from build123d import *

# Parameters (mm, degrees)
F0_W     = 125
F0_H     = 100
F2_DEPTH = 63.5
F1_R     = 37.5
F3_DEPTH = 2.5
F5_DEPTH = 1
F6_R     = 1.5
F7_DEPTH = 20


# Not quite as in the source:
# - a feature names something its author has since deleted; it is built from what else it names


with BuildPart() as f2:
    # F0 (on Front) → F2 (new body)
    with BuildSketch(Plane.XZ):
        with Locations((0, 17.5)):
            Rectangle(F0_W, F0_H)
    extrude(amount=-F2_DEPTH)

    # F1 (on Front) → F3 (cut, symmetric)
    with BuildSketch(Plane.XZ):
        with Locations((-13.5, 22.6666666667)):
            Circle(F1_R)
    extrude(amount=F3_DEPTH, both=True, mode=Mode.SUBTRACT)

    # F4 (on face) → F5 (cut)
    with BuildSketch(Plane.XY.offset(67.5)):
        Polygon((51.0344103292, 5), (52.5, 5), (52.5, 7.5384757729), align=None)
        Polygon((46.0344103292, 5), (51.0344103292, 5), (52.5, 7.5384757729), (52.5, 16.1987298108), align=None)
        Polygon((36.0344103292, 5), (41.0344103292, 5), (52.5, 24.8589838486), (52.5, 33.5192378865), align=None)
        Polygon((26.0344103292, 5), (31.0344103292, 5), (52.5, 42.1794919243), (52.5, 50.8397459622), align=None)
        Polygon((16.0344103292, 5), (21.0344103292, 5), (52.5, 59.5), (47.5, 59.5), align=None)
        Polygon((-32.5, 59.5), (-52.5, 24.8589838486), (-52.5, 16.1987298108), (-27.5, 59.5), align=None)
        Polygon((6.0344103292, 5), (11.0344103292, 5), (42.5, 59.5), (37.5, 59.5), align=None)
        Polygon((-52.5, 42.1794919243), (-52.5, 33.5192378865), (-37.5, 59.5), (-42.5, 59.5), align=None)
        Polygon((-47.5, 59.5), (-52.5, 59.5), (-52.5, 50.8397459622), align=None)
        Polygon((-22.5, 59.5), (-52.5, 7.5384757729), (-52.5, 5), (-48.9655896708, 5), (-17.5, 59.5), align=None)
        Polygon((-3.9655896708, 5), (1.0344103292, 5), (32.5, 59.5), (27.5, 59.5), align=None)
        Polygon((-13.9655896708, 5), (-8.9655896708, 5), (22.5, 59.5), (17.5, 59.5), align=None)
        Polygon((-12.5, 59.5), (-43.9655896708, 5), (-38.9655896708, 5), (-7.5, 59.5), align=None)
        Polygon((-23.9655896708, 5), (-18.9655896708, 5), (12.5, 59.5), (7.5, 59.5), align=None)
        Polygon((-2.5, 59.5), (-33.9655896708, 5), (-28.9655896708, 5), (2.5, 59.5), align=None)
    extrude(amount=-F5_DEPTH, mode=Mode.SUBTRACT)

    # F6 (on face) → F7 (cut)
    with BuildSketch(Plane.XY.offset(67.5)):
        with Locations((-56.5, 57.5)):
            Circle(F6_R)
        with Locations((56.5, 57.5)):
            Circle(F6_R)
        with Locations((56.5, 6)):
            Circle(F6_R)
        with Locations((-56.5, 6)):
            Circle(F6_R)
    extrude(amount=-F7_DEPTH, mode=Mode.SUBTRACT)


solid = f2.part
The model under review builds one solid part; all positions refer to its coordinate system, in mm. Coordinates: 2 decimals unless noted, no trailing zeros. Loops run counter-clockwise (first coordinate to the right, second up) from the corner with the lowest first, then second, coordinate; pieces in that order, holes last.
(1) Consider section B-B, the plane z = 35. Give the boundary of the cut face in (x, y).
Determined:
outline: (-62.5, 0) - (-48.91, 0) - (-48.91, 2.5) - (21.91, 2.5) - (21.91, 0) - (62.5, 0) - (62.5, 63.5) - (-62.5, 63.5) - close
(2) Wall thickness on L1, parallel to Y at x = -56.5, z = 63.5; L2, parallel to Y at x = -56, z = 55; L3, parallel to Y at x = -42.5, z = 9: over which ranges is each line inside the solid? List them lowest first.
Determined:
L1: y = 0 to 4.5, 7.5 to 56, 59 to 63.5
L2: y = 0 to 4.59, 7.41 to 56.09, 58.91 to 63.5
L3: y = 2.5 to 63.5
(3) Consider section A-A, the plane x = 56.5. Give the boundary of the cut face in (y, z).
Determined:
outline: (0, -32.5) - (63.5, -32.5) - (63.5, 67.5) - (59, 67.5) - (59, 47.5) - (56, 47.5) - (56, 67.5) - (7.5, 67.5) - (7.5, 47.5) - (4.5, 47.5) - (4.5, 67.5) - (0, 67.5) - close
(4) Insertion check: P1, Ø3.5, axis at x = 57, y = 57, coming from the +Z side; P2, Ø3, axis at x = 0, z = 48.5, coming from the -Y side; P3, Ø2.5, axis at x = 56.5, y = 6, coming from the +Z side; P4, Ø1, axis at x = -49, y = 11.5, coming from the +Z side. Each pin has a flat end and moves straight along its axis. Give the tip position at first contact, or say it passes through.
Determined:
P1: stops at z = 67.5
P2: stops at y = 2.5
P3: stops at z = 47.5
P4: stops at z = 66.5
(5) Draft analysis for pull direction Y (two halves, no side actions). For faces 1 (the flat face through (-14, 2.5, 23)), 2 (the flat face through (41.6, 23.3, 67)), 3 (the flat face through (-41, 41, 66.5)), 4 (the flat face through (-1, 31, 67.5)), state which applies: +Y half, -Y half, draft (parallel to the pull), parting line (faces both ways), or undercut.
Determined:
face 1: -Y half
face 2: undercut
face 3: undercut
face 4: draft
(6) Consider section C-C, the plane z = 19. Give the boundary of the cut face in (x, y).
Determined:
outline: (-62.5, 0) - (-50.82, 0) - (-50.82, 2.5) - (23.82, 2.5) - (23.82, 0) - (62.5, 0) - (62.5, 63.5) - (-62.5, 63.5) - close
